Verification items for the finished model (mm, model axes). Coordinates: 2 decimals unless noted, no trailing zeros. Write each loop counter-clockwise with the first axis right and the second up, starting at its lowest first coordinate (ties: lowest second). Pieces come first, ordered by that corner, then holes. Notation, with made-up numbers: (76, 76.25) - (103, 76.25) arc R20 cw to (103, 81.25) - close; hole circle Ø5 at (60, 13). An arc over 180 degrees is marked (long way). Use CSV: the item, a comma, the result in double quotes. Start each with the question number.
```python
from build123d import *

# Parameters (mm, degrees)
F0_R     = 2.5
F0_R_2   = 4
F1_DEPTH = 5
F0_W     = 6
F0_H     = 8
F2_DEPTH = 7
F3_SIZE  = 1
F4_DEPTH = 5
F5_SIZE  = 2


with BuildPart() as f1:
    # F0 (on Top) → F1 (new body)
    with BuildSketch(Plane.XY):
        Polygon((-77.5, 15), (-84.5, 15), (-84.5, -15), (-77.5, -15), (-77.5, -7), (-71.5, -7), (-71.5, -15), (71.5, -15), (71.5, -7), (77.5, -7), (77.5, -15), (84.5, -15), (84.5, 15), (77.5, 15), (77.5, 7), (71.5, 7), (71.5, 15), (-71.5, 15), (-71.5, 7), (-77.5, 7), align=None)
        with Locations((-30, -7.5)):
            Circle(F0_R, mode=Mode.SUBTRACT)
        with Locations((30, -7.5)):
            Circle(F0_R, mode=Mode.SUBTRACT)
        with Locations((-74.5, 0)):
            Circle(F0_R, mode=Mode.SUBTRACT)
        with Locations((-43, 0)):
            Circle(F0_R_2, mode=Mode.SUBTRACT)
        with Locations((-30, 7.5)):
            Circle(F0_R, mode=Mode.SUBTRACT)
        with Locations((43, 0)):
            Circle(F0_R_2, mode=Mode.SUBTRACT)
        with Locations((74.5, 0)):
            Circle(F0_R, mode=Mode.SUBTRACT)
        with Locations((30, 7.5)):
            Circle(F0_R, mode=Mode.SUBTRACT)
        with Locations((-43, 0)):
            Circle(F0_R_2)
        with Locations((-43, 0)):
            Circle(F0_R, mode=Mode.SUBTRACT)
        with Locations((43, 0)):
            Circle(F0_R_2)
        with Locations((43, 0)):
            Circle(F0_R, mode=Mode.SUBTRACT)
    extrude(amount=F1_DEPTH)

    # F0 (on Top) → F2 (join)
    with BuildSketch(Plane.XY):
        with Locations((-74.5, 11)):
            Rectangle(F0_W, F0_H)
        with Locations((-74.5, -11)):
            Rectangle(F0_W, F0_H)
        with Locations((74.5, -11)):
            Rectangle(F0_W, F0_H)
        with Locations((74.5, 11)):
            Rectangle(F0_W, F0_H)
    extrude(amount=F2_DEPTH)

    # F3
    f3_edges = [f1.edges().sort_by_distance(p)[0] for p in [
        (-77.5, 11, 7),
        (-71.5, 11, 7),
        (-74.5, 7, 7),
        (-74.5, -7, 7),
        (-71.5, -11, 7),
        (-77.5, -11, 7),
        (77.5, 11, 7),
        (74.5, 7, 7),
        (71.5, 11, 7),
        (74.5, -7, 7),
        (77.5, -11, 7),
        (71.5, -11, 7),
    ]]
    chamfer(f3_edges, length=F3_SIZE)

    # F0 (on Top) → F4 (join)
    with BuildSketch(Plane.XY):
        with Locations((43, 0)):
            Circle(F0_R_2)
        with Locations((43, 0)):
            Circle(F0_R, mode=Mode.SUBTRACT)
        with Locations((-43, 0)):
            Circle(F0_R_2)
        with Locations((-43, 0)):
            Circle(F0_R, mode=Mode.SUBTRACT)
    extrude(amount=-F4_DEPTH)

    # F5
    f5_edges = [f1.edges().sort_by_distance(p)[0] for p in [
        (-84.5, -15, 2.5),
        (-84.5, 15, 2.5),
        (84.5, -15, 2.5),
        (84.5, 15, 2.5),
    ]]
    chamfer(f5_edges, length=F5_SIZE)


solid = f1.part
```
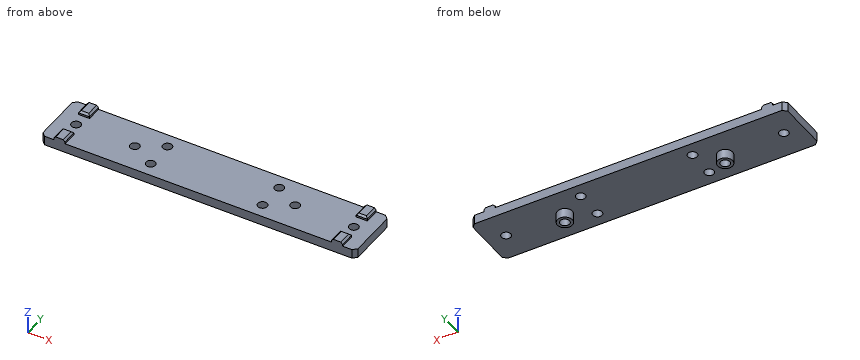
Q1. Cross-section at B-B (z = 3.5). State how many separate pieces and enclosed holes the cut face has, plus the area to 3 significant figures.
Q2. Gauge pin test, flat ends, axial feed: pin 1 (0.5 mm diameter, centred on y = 10.5, z = 5.5, fed in from -X); pin 2 (3 mm diameter, centred on x = 43, y = 0, fed in from -Z); pin 3 (12 mm diameter, centred on x = 54.5, y = 9.5, fed in from -Z); pin 4 (2 mm diameter, centred on y = -3, z = -1.5, fed in from +X). Record the tip position at first contact, or that the pin passes through.
Q3. Cross-section at A-A (x = 74.5). Record the cut outline in (y, z).
Q4. Cross-section at C-C (x = 43). Record the cut outline in (y, z).
Q5. Scan lines: line 1 along Y through (x, z) = (-30, 1.45); line 2 along Y through (x, z) = (43, -0.5); line 3 along X through (y, z) = (-5.5, 1.5). Record each from-to range of solid material in increasing order. Write a range as from..to.
Reply:
1,separate pieces,"1"
1,enclosed holes,"8"
1,area,"4,900 mm^2"
2,pin 1,"x = -77.5"
2,pin 2,"through"
2,pin 3,"z = 0"
2,pin 4,"x = 46.46"
3,outline,"(-15, 0) - (-2.5, 0) - (-2.5, 5) - (-7, 5) - (-7, 6) - (-8, 7) - (-15, 7) - close; (2.5, 0) - (15, 0) - (15, 7) - (8, 7) - (7, 6) - (7, 5) - (2.5, 5) - close"
4,outline,"(-15, 0) - (-4, 0) - (-4, -5) - (-2.5, -5) - (-2.5, 5) - (-15, 5) - close; (2.5, -5) - (4, -5) - (4, 0) - (15, 0) - (15, 5) - (2.5, 5) - close"
5,line 1,"-15..-10, -5..5, 10..15"
5,line 2,"-4..-2.5, 2.5..4"
5,line 3,"-84.5..-31.5, -28.5..28.5, 31.5..84.5"
